Geometry check sheet. Reference: drawing and pictorial views, mm from the part's lowest x, y, z. A direction names the side the tool comes from. Give positions to 0.01 mm unless a question says otherwise; leave off trailing zeros. Write each loop counter-clockwise with the first axis right and the second up, starting at its lowest first coordinate (ties: lowest second). Pieces come first, ordered by that corner, then holes. Notation, with made-up numbers: (-13.75, -2.75) -> (27.25, -2.75) arc R24 cw to (27.25, 23.25) -> close; hole circle Ø2 at (55.5, 25.5). An arc over 180 degrees is marked (long way). Return JSON: item names as keys, results as strings.
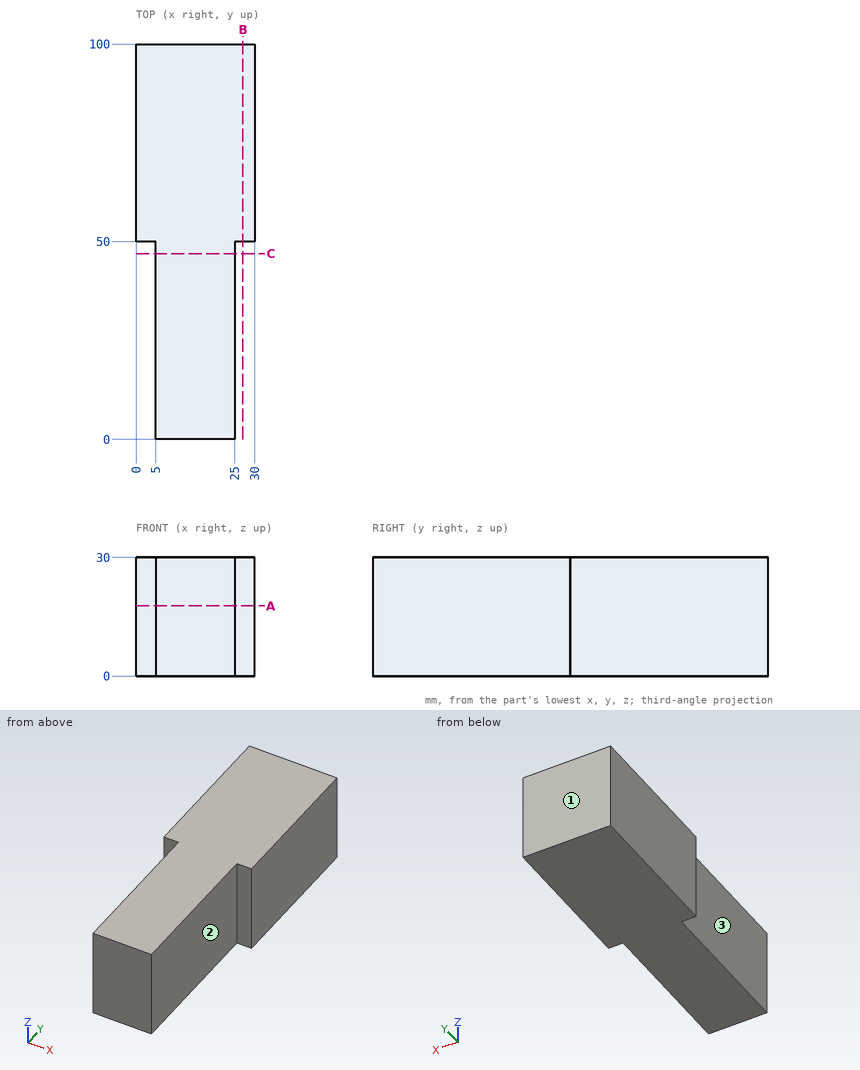
(1) Thickness scan on L1, parallel to X at y = 30.5, z = 14; L2, parallel to Y at x = 26, z = 3. Record the ranges inside material, lowest first.
Reply:
{"L1": "5 to 25", "L2": "50 to 100"}
(2) Cross-section at A-A on z = 17.75. Enter the section's corners in (x, y).
Reply:
{"outline": "(0, 50) -> (5, 50) -> (5, 0) -> (25, 0) -> (25, 50) -> (30, 50) -> (30, 100) -> (0, 100) -> close"}
(3) Set-up check for the marked faces 1, 2 and 3: record each of +Z, -Z, +X, -X, +Y, -Y from which the full face is reachable in a straight line by a thin tool's end or side.
Reply:
{"face 1": "+Z, -Z, +X, -X, +Y", "face 2": "+Z, -Z, +X, -Y", "face 3": "+Z, -Z, -X, -Y"}
(4) Cross-section at B-B on x = 27. Enter the section's corners in (y, z), then the cut area to 3 significant figures.
Reply:
{"outline": "(50, 0) -> (100, 0) -> (100, 30) -> (50, 30) -> close", "area": "1,500 mm^2"}
(5) Cross-section at C-C on y = 47. Enter the section's corners in (x, z), then the cut area to 3 significant figures.
Reply:
{"outline": "(5, 0) -> (25, 0) -> (25, 30) -> (5, 30) -> close", "area": "600 mm^2"}
(6) Depth check by flat-ended pin: pin 1 Ø3 at (y, z) = (32.5, 23.5) entering from -X; pin 2 Ø2.5 at (x, z) = (26.5, 8.5) entering from -Y. Enter the tip coordinate at first touch or a pass-through.
Reply:
{"pin 1": "x = 5", "pin 2": "y = 50"}
